Model file for the job. Use its own axes, mm. Face numbers are marked on the shaded views. Give positions to 0.01 mm unless a question says otherwise; leave off trailing zeros. Order: outer loops, then holes, each group sorted by start corner. A loop starts at its lowest first (then second) coordinate and runs counter-clockwise, first axis right, second up. Notation, with made-up numbers: (-28, -2.5) - (30, -2.5) arc R25 cw to (30, 19.5) - close; hole circle Ø6 at (-37.5, -2). An arc over 180 degrees is marked (long way). Return JSON: item names as keys, results as strings. Group by question number.
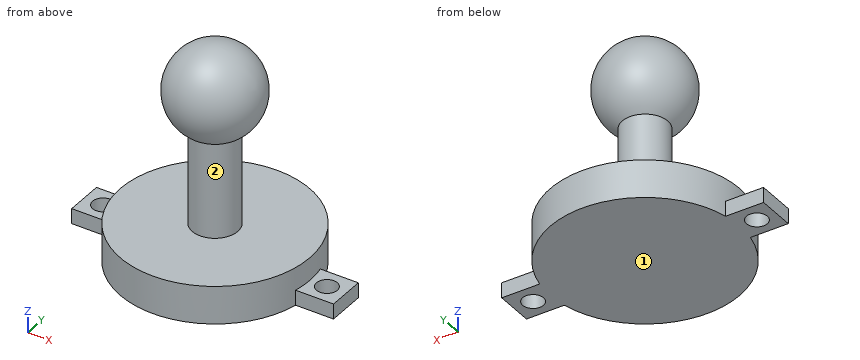
from build123d import *

# Parameters (mm, degrees)
F2_W     = 10
F2_H     = 10
F2_R     = 2.75
F3_DEPTH = 4


# Not quite as in the source:
# - a pattern or mirror of a feature is missing from the dataset's text; its kind, count and spacing are read off the source's solid


with BuildPart() as f1:
    # F0 (on Front) → F1 (revolve)
    with BuildSketch(Plane.XZ):
        with BuildLine():
            Line((25, 10), (6, 10))
            Line((6, 10), (6, 35))
            ThreePointArc((6, 35), (11.5911099155, 48.4981333866), (0, 57.3923048454))
            Line((0, 57.3923048454), (0, 0))
            Line((0, 0), (25, 0))
            Line((25, 0), (25, 10))
        make_face()
    revolve(axis=Axis((0, 0, 28.6961524227), (0, 0, -1)))

    # F2 (on face) → F3 (join)
    with BuildSketch(Plane(origin=(0, 0, 0), x_dir=(1, 0, 0), z_dir=(0, 0, -1))):
        with Locations((29.4948974278, 0)):
            Rectangle(F2_W, F2_H)
        with Locations((29.4948974278, 0)):
            Circle(F2_R, mode=Mode.SUBTRACT)
    f3 = extrude(amount=-F3_DEPTH)

    # F3_copies: F3 across plane
    add(f3.mirror(Plane(origin=(0, 0, 0), x_dir=(0, 0, -1), z_dir=(-1, 0, 0))))


solid = f1.part
(1) Slice it at A-A (y = 0). Give the cut face in (x, z).
(2) Drill centre lines: L1, parallel to X at y = 0, z = 2; L2, parallel to Z at x = -18, y = -5; L3, parallel to Z at x = 3, y = -8. Where is each one in solid material? Low to high.
(3) Drop flat-ended pins along their axis: pin 1 Ø2 at (x, y) = (-17, 11) entering from -Z; pin 2 Ø1.2 at (x, z) = (-31.5, 2) entering from -Y; pin 3 Ø2 at (x, z) = (-31, 2) entering from +Y; pin 4 Ø5 at (x, z) = (9, 38.5) entering from -Y. Give the stop position or say it passes through.
(4) Slice it at C-C (z = 23.5). Give the cut face in (x, y), and give its area (3 significant figures).
(5) Slice it at B-B (x = 3). Give the cut face in (y, z).
(6) Slice it at D-D (y = -16). Give the cut face in (x, z).
(7) Pull direction Z, two halves, no side cores. Call the marked faces 1 and 2: released by +Z, released by -Z, zero draft, split by the parting line, or undercut.
Result set:
{
 "1": {"outline": "(-34.49, 0) - (-32.24, 0) - (-32.24, 4) - (-34.49, 4) - close; (-26.74, 0) - (26.74, 0) - (26.74, 4) - (25, 4) - (25, 10) - (6, 10) - (6, 35) arc R12 ccw (long way) to (-6, 35) - (-6, 10) - (-25, 10) - (-25, 4) - (-26.74, 4) - close; (32.24, 0) - (34.49, 0) - (34.49, 4) - (32.24, 4) - close"},
 "2": {"L1": "x = -34.49 to -32.24, -26.74 to 26.74, 32.24 to 34.49", "L2": "z = 0 to 10", "L3": "z = 0 to 10, 36.97 to 53.82"},
 "3": {"pin 1": "stops at z = 0", "pin 2": "stops at y = -5", "pin 3": "stops at y = 5", "pin 4": "stops at y = -8.12"},
 "4": {"outline": "circle Ø12 at (0, 0)", "area": "113 mm²"},
 "5": {"outline": "(-24.82, 0) - (24.82, 0) - (24.82, 10) - (5.2, 10) - (5.2, 35) arc R11.62 ccw (long way) to (-5.2, 35) - (-5.2, 10) - (-24.82, 10) - close"},
 "6": {"outline": "(-19.21, 0) - (19.21, 0) - (19.21, 10) - (-19.21, 10) - close"},
 "7": {"face 1": "released by -Z", "face 2": "undercut"}
}
